```python
from build123d import *

# Parameters (mm, degrees)
SKETCH1_W           = 247.65
SKETCH1_H           = 63.5
BOSS_EXTRUDE1_DEPTH = 76.2
CUT_EXTRUDE1_DEPTH  = 57.15
SKETCH5_R           = 2.159
CUT_EXTRUDE3_DEPTH  = 6.35
SKETCH7_R           = 5.08
CUT_EXTRUDE5_DEPTH  = 25.4
FILLET1_R           = 12.7
CUT_EXTRUDE6_DEPTH  = 2.54
SKETCH9_R           = 3.302
CUT_EXTRUDE7_DEPTH  = 12.7


with BuildPart() as part:
    # Sketch1 → Boss-Extrude1 (new body)
    with BuildSketch(Plane(origin=(0, 0, 0), x_dir=(1, 0, 0), z_dir=(0, 1, 0))):
        Rectangle(SKETCH1_W, SKETCH1_H)
    extrude(amount=BOSS_EXTRUDE1_DEPTH)

    # Sketch2 → Cut-Extrude1 (cut)
    with BuildSketch(Plane.XY.offset(31.75)):
        with BuildLine():
            Line((-88.9, 55.88), (88.9, 55.88))
            ThreePointArc((88.9, 55.88), (106.68, 38.1), (88.9, 20.32))
            Line((88.9, 20.32), (-88.9, 20.32))
            ThreePointArc((-88.9, 20.32), (-106.68, 38.1), (-88.9, 55.88))
        make_face()
    extrude(amount=-CUT_EXTRUDE1_DEPTH, mode=Mode.SUBTRACT)

    # Sketch5 → Cut-Extrude3 (cut)
    with BuildSketch(Plane.XY.offset(31.75)):
        with Locations((0, 69.85)):
            Circle(SKETCH5_R)
        with Locations((33.02, 69.85)):
            Circle(SKETCH5_R)
        with Locations((66.04, 69.85)):
            Circle(SKETCH5_R)
        with Locations((-66.04, 69.85)):
            Circle(SKETCH5_R)
        with Locations((-33.02, 69.85)):
            Circle(SKETCH5_R)
        with Locations((-99.06, 69.85)):
            Circle(SKETCH5_R)
        with Locations((99.06, 69.85)):
            Circle(SKETCH5_R)
        with Locations((-99.06, 6.35)):
            Circle(SKETCH5_R)
        with Locations((-66.04, 6.35)):
            Circle(SKETCH5_R)
        with Locations((-33.02, 6.35)):
            Circle(SKETCH5_R)
        with Locations((0, 6.35)):
            Circle(SKETCH5_R)
        with Locations((33.02, 6.35)):
            Circle(SKETCH5_R)
        with Locations((66.04, 6.35)):
            Circle(SKETCH5_R)
        with Locations((99.06, 6.35)):
            Circle(SKETCH5_R)
        with Locations((-117.475, 50.8)):
            Circle(SKETCH5_R)
        with Locations((117.475, 50.8)):
            Circle(SKETCH5_R)
        with Locations((-117.475, 25.4)):
            Circle(SKETCH5_R)
        with Locations((117.475, 25.4)):
            Circle(SKETCH5_R)
    extrude(amount=-CUT_EXTRUDE3_DEPTH, mode=Mode.SUBTRACT)

    # Sketch7 → Cut-Extrude5 (cut)
    with BuildSketch(Plane(origin=(0, 0, 0), x_dir=(-1, 0, 0), z_dir=(0, -1, 0))):
        with Locations((-83.185, 15.24)):
            Circle(SKETCH7_R)
    extrude(amount=-CUT_EXTRUDE5_DEPTH, mode=Mode.SUBTRACT)

    # Fillet1
    fillet1_edges = [part.edges().sort_by_distance(p)[0] for p in [
        (-123.825, 0, 0),
        (123.825, 0, 0),
    ]]
    fillet(fillet1_edges, radius=FILLET1_R)

    # Sketch8 → Cut-Extrude6 (cut)
    with BuildSketch(Plane.XY.offset(31.75)):
        with BuildLine():
            Line((-88.9, 13.97), (88.9, 13.97))
            ThreePointArc((88.9, 13.97), (113.03, 38.1), (88.9, 62.23))
            Line((88.9, 62.23), (-88.9, 62.23))
            ThreePointArc((-88.9, 62.23), (-113.03, 38.1), (-88.9, 13.97))
        make_face()
        with BuildLine():
            ThreePointArc((88.9, 16.51), (110.49, 38.1), (88.9, 59.69))
            Line((88.9, 59.69), (-88.9, 59.69))
            ThreePointArc((-88.9, 59.69), (-110.49, 38.1), (-88.9, 16.51))
            Line((-88.9, 16.51), (88.9, 16.51))
        make_face(mode=Mode.SUBTRACT)
    extrude(amount=-CUT_EXTRUDE6_DEPTH, mode=Mode.SUBTRACT)

    # Sketch9 → Cut-Extrude7 (cut)
    with BuildSketch(Plane(origin=(0, 76.2, 44.45), x_dir=(-1, 0, 0), z_dir=(0, -1, 0))):
        with Locations((-111.125, 63.5)):
            Circle(SKETCH9_R)
        with Locations((-66.675, 63.5)):
            Circle(SKETCH9_R)
        with Locations((-22.225, 63.5)):
            Circle(SKETCH9_R)
        with Locations((22.225, 63.5)):
            Circle(SKETCH9_R)
        with Locations((66.675, 63.5)):
            Circle(SKETCH9_R)
        with Locations((111.125, 63.5)):
            Circle(SKETCH9_R)
    extrude(amount=CUT_EXTRUDE7_DEPTH, mode=Mode.SUBTRACT)


solid = part.part
```
Read the model definition and answer for the solid it produces. Units are mm, in the model's axes. A direction names the side the tool comes from. Give positions to 0.01 mm unless a question says otherwise; leave off trailing zeros. Order: outer loops, then holes, each group sorted by start corner. A loop starts at its lowest first (then second) coordinate and runs counter-clockwise, first axis right, second up.
(1) For faces 1 (the flat face through (-99, 6, 25.4)), 2 (the cylindrical face through (84.29, 10.02, -10.28)), 3 (the cylindrical face through (-69.725, 69.939, -17.785)), 4 (the flat face through (-2, 38, -31.75)), determine the directions among +Z, -Z, +X, -X, +Y, -Y from which every point of the face is accessible in a straight line to the end or side of a thin tool.
(2) Find section D-D (x = 99.06). Give the vertices of the cut face in (y, z).
(3) Given pin 1 (3.5 mm diameter, centred on x = 22, z = -18.5, fed in from +Y); pin 2 (3.5 mm diameter, centred on x = 117.5, y = 50.5, fed in from +Z), each flat-ended and moving along its own axis, determine where each tip first touches the part or whether it passes through.
(4) Find section B-B (x = 0). Give the vertices of the cut face in (y, z).
(5) Straight lines are drawn through the part: L1, parallel to Y at x = -33.02, z = 28.75; L2, parallel to Y at x = -12, z = 14.5; L3, parallel to Z at x = 1, y = 52. For each, find the intervals that lie inside material, in ascending order.
(6) For a pull along Y with two mould halves and no side action, classify faces 5 (the flat face through (-118, 25, 25.4)), 6 (the cylindrical face through (65.15, 69.94, -16.12)), 7 (the flat face through (-22, 63.5, -19)), 8 (the cylindrical face through (-63.98, 7, 28.62)) as released by +Y, released by -Y, zero draft, split by the parting line, or undercut.
(7) Find section A-A (y = 38.1). Give the vertices of the cut face in (x, z) (3 decimals).
(8) Find section C-C (y = 69.85). Give the number of separate pieces and of enclosed holes in the cut face, plus the area to 3 significant figures.
Result sheet:
1. face 1: +Z
1. face 2: -Y
1. face 3: +Y
1. face 4: -Z, +X, -X, +Y, -Y
2. outline: (0, -31.75) - (76.2, -31.75) - (76.2, 31.75) - (72.01, 31.75) - (72.01, 25.4) - (67.69, 25.4) - (67.69, 31.75) - (59.99, 31.75) - (59.99, 29.21) - (57.15, 29.21) - (57.15, 31.75) - (52.69, 31.75) - (52.69, -25.4) - (23.51, -25.4) - (23.51, 31.75) - (19.05, 31.75) - (19.05, 29.21) - (16.21, 29.21) - (16.21, 31.75) - (8.51, 31.75) - (8.51, 25.4) - (4.19, 25.4) - (4.19, 31.75) - (0, 31.75) - close
3. pin 1: stops at y = 63.5
3. pin 2: stops at z = 25.4
4. outline: (0, -31.75) - (76.2, -31.75) - (76.2, 31.75) - (72.01, 31.75) - (72.01, 25.4) - (67.69, 25.4) - (67.69, 31.75) - (62.23, 31.75) - (62.23, 29.21) - (59.69, 29.21) - (59.69, 31.75) - (55.88, 31.75) - (55.88, -25.4) - (20.32, -25.4) - (20.32, 31.75) - (16.51, 31.75) - (16.51, 29.21) - (13.97, 29.21) - (13.97, 31.75) - (8.51, 31.75) - (8.51, 25.4) - (4.19, 25.4) - (4.19, 31.75) - (0, 31.75) - close
5. L1: y = 0 to 4.19, 8.51 to 20.32, 55.88 to 67.69, 72.01 to 76.2
5. L2: y = 0 to 20.32, 55.88 to 76.2
5. L3: z = -31.75 to -25.4
6. face 5: undercut
6. face 6: zero draft
6. face 7: released by +Y
6. face 8: undercut
7. outline: (-123.825, -31.75) - (123.825, -31.75) - (123.825, 31.75) - (113.03, 31.75) - (113.03, 29.21) - (110.49, 29.21) - (110.49, 31.75) - (106.68, 31.75) - (106.68, -25.4) - (-106.68, -25.4) - (-106.68, 31.75) - (-110.49, 31.75) - (-110.49, 29.21) - (-113.03, 29.21) - (-113.03, 31.75) - (-123.825, 31.75) - close
8. separate pieces: 1
8. enclosed holes: 6
8. area: 15,300 mm2
